Check sheet for the modelled part. Datum: model origin and axes. Units: mm. A direction names the side the tool comes from. Give positions to 0.01 mm unless a question says otherwise; leave off trailing zeros. Write each loop counter-clockwise with the first axis right and the second up, starting at its lowest first coordinate (ties: lowest second). Pieces come first, ordered by that corner, then holes. Notation, with made-up numbers: (67, 10) -> (81, 10) arc R27 cw to (81, 29) -> close; hole circle Ø3 at (4.5, 16.5). An arc over 180 degrees is marked (long way). Answer as a JSON object with one key per item and string values.
from build123d import *

# Parameters (mm, degrees)
F0_W          = 125
F0_H          = 40
F0_R          = 5
F1_DEPTH      = 25
F2_R          = 11
F3_DEPTH      = 10
F4_W          = 40
F4_H          = 25
F5_DEPTH      = 25
F6_R          = 4.25
F7_DEPTH      = 40
F9_DEPTH      = 6
F10_T4_DEPTH  = 25
F10_T10_DEPTH = 25
F10_T16_DEPTH = 25
F10_T23_DEPTH = 25
F10_T29_DEPTH = 25
F10_T35_DEPTH = 25
F10_T41_DEPTH = 25
F10_T47_DEPTH = 25
F10_T54_DEPTH = 25
F10_T60_DEPTH = 25
F10_T63_DEPTH = 50


# Not quite as in the source:
# - a fillet or chamfer that OpenCascade refuses, or shapes differently, is made with other operations: its cross-section is extruded or revolved along the edge and cut away or added


with BuildPart() as f1:
    # F0 (on Front) → F1 (new body)
    with BuildSketch(Plane.XZ):
        with Locations((-7.5, 0)):
            Rectangle(F0_W, F0_H)
        with Locations((-50, 0)):
            Circle(F0_R, mode=Mode.SUBTRACT)
        Circle(F0_R, mode=Mode.SUBTRACT)
        with Locations((40, 0)):
            Circle(F0_R, mode=Mode.SUBTRACT)
    extrude(amount=F1_DEPTH)

    # F2 (on face) → F3 (cut)
    with BuildSketch(Plane.XZ.offset(25)):
        with Locations((-50, 0)):
            Circle(F2_R)
        Circle(F2_R)
        with Locations((40, 0)):
            Circle(F2_R)
    extrude(amount=-F3_DEPTH, mode=Mode.SUBTRACT)

    # F4 (on face) → F5 (join)
    with BuildSketch(Plane(origin=(0, 0, 0), x_dir=(-1, 0, 0), z_dir=(0, 1, 0))):
        with Locations((50, 32.5)):
            Rectangle(F4_W, F4_H)
        with Locations((50, -32.5)):
            Rectangle(F4_W, F4_H)
    extrude(amount=-F5_DEPTH)

    # F6 (on face) → F7 (cut, through all)
    with BuildSketch(Plane(origin=(-70, 0, 0), x_dir=(0, -1, 0), z_dir=(-1, 0, 0))):
        with Locations((12.5, 27.5)):
            Circle(F6_R)
        with Locations((12.5, -27.5)):
            Circle(F6_R)
    extrude(amount=-F7_DEPTH, mode=Mode.SUBTRACT)

    # F8 (on face) → F9 (cut)
    with BuildSketch(Plane.YZ.offset(-30)):
        Polygon((-8.4585481157, 34.5), (-16.5414518843, 34.5), (-20.5829037687, 27.5), (-16.5414518843, 20.5), (-8.4585481157, 20.5), (-4.4170962313, 27.5), align=None)
        Polygon((-8.4585481157, -20.5), (-16.5414518843, -20.5), (-20.5829037687, -27.5), (-16.5414518843, -34.5), (-8.4585481157, -34.5), (-4.4170962313, -27.5), align=None)
    extrude(amount=-F9_DEPTH, mode=Mode.SUBTRACT)

    # F10: fillet of radius 5 on 6 edges, made by hand


with BuildPart() as f10_tool2:
    # F10_s3 → F10_t4 (new body)
    with BuildSketch(Plane.XZ):
        with BuildLine():
            ThreePointArc((-25, 20), (-28.5355339059, 21.4644660941), (-30, 25))
            Line((-30, 25), (-30, 20))
            Line((-30, 20), (-25, 20))
        make_face()
    extrude(amount=F10_T4_DEPTH)

    split(bisect_by=Plane.XY.offset(20.5), keep=Keep.BOTTOM)

    split(bisect_by=Plane(origin=(0, -15.2206714755, 8.7876587737), x_dir=(1, 0, 0), z_dir=(0, 0.8660254038, -0.5)), keep=Keep.TOP)


with BuildPart() as f1_1:
    add(f1.part)

    # F10_t1: union F10_tool2
    add(f10_tool2.part)


with BuildPart() as f10_tool8:
    # F10_s9 → F10_t10 (new body)
    with BuildSketch(Plane.XZ):
        with BuildLine():
            ThreePointArc((-25, 20), (-28.5355339059, 21.4644660941), (-30, 25))
            Line((-30, 25), (-30, 20))
            Line((-30, 20), (-25, 20))
        make_face()
    extrude(amount=F10_T10_DEPTH)

    split(bisect_by=Plane.XY.offset(20.5), keep=Keep.TOP)

    split(bisect_by=Plane(origin=(0, -15.2206714755, 8.7876587737), x_dir=(1, 0, 0), z_dir=(0, 0.8660254038, -0.5)), keep=Keep.TOP)


with BuildPart() as f1_2:
    add(f1_1.part)

    # F10_t7: union F10_tool8
    add(f10_tool8.part)


with BuildPart() as f10_tool14:
    # F10_s15 → F10_t16 (new body)
    with BuildSketch(Plane.XZ):
        with BuildLine():
            ThreePointArc((-25, 20), (-28.5355339059, 21.4644660941), (-30, 25))
            Line((-30, 25), (-30, 20))
            Line((-30, 20), (-25, 20))
        make_face()
    extrude(amount=F10_T16_DEPTH)

    split(bisect_by=Plane(origin=(0, -3.5293285245, -2.0376587737), x_dir=(1, 0, 0), z_dir=(0, 0.8660254038, 0.5)), keep=Keep.TOP)

    split(bisect_by=Plane.XY.offset(20.5), keep=Keep.BOTTOM)

    split(bisect_by=Plane(origin=(0, -15.2206714755, 8.7876587737), x_dir=(1, 0, 0), z_dir=(0, -0.8660254038, 0.5)), keep=Keep.TOP)


with BuildPart() as f1_3:
    add(f1_2.part)

    # F10_t13: union F10_tool14
    add(f10_tool14.part)


with BuildPart() as f10_tool21:
    # F10_s22 → F10_t23 (new body)
    with BuildSketch(Plane.XZ):
        with BuildLine():
            ThreePointArc((-25, 20), (-28.5355339059, 21.4644660941), (-30, 25))
            Line((-30, 25), (-30, 20))
            Line((-30, 20), (-25, 20))
        make_face()
    extrude(amount=F10_T23_DEPTH)

    split(bisect_by=Plane(origin=(0, -3.5293285245, -2.0376587737), x_dir=(1, 0, 0), z_dir=(0, -0.8660254038, -0.5)), keep=Keep.TOP)

    split(bisect_by=Plane.XY.offset(20.5), keep=Keep.BOTTOM)


with BuildPart() as f1_4:
    add(f1_3.part)

    # F10_t20: union F10_tool21
    add(f10_tool21.part)


with BuildPart() as f10_tool27:
    # F10_s28 → F10_t29 (new body)
    with BuildSketch(Plane.XZ):
        with BuildLine():
            ThreePointArc((-25, 20), (-28.5355339059, 21.4644660941), (-30, 25))
            Line((-30, 25), (-30, 20))
            Line((-30, 20), (-25, 20))
        make_face()
    extrude(amount=F10_T29_DEPTH)

    split(bisect_by=Plane(origin=(0, -3.5293285245, -2.0376587737), x_dir=(1, 0, 0), z_dir=(0, -0.8660254038, -0.5)), keep=Keep.TOP)

    split(bisect_by=Plane.XY.offset(20.5), keep=Keep.TOP)


with BuildPart() as f1_5:
    add(f1_4.part)

    # F10_t26: union F10_tool27
    add(f10_tool27.part)


with BuildPart() as f10_tool33:
    # F10_s34 → F10_t35 (new body)
    with BuildSketch(Plane.XZ):
        with BuildLine():
            ThreePointArc((-25, -20), (-28.5355339059, -21.4644660941), (-30, -25))
            Line((-30, -25), (-30, -20))
            Line((-30, -20), (-25, -20))
        make_face()
    extrude(amount=F10_T35_DEPTH)

    split(bisect_by=Plane.XY.offset(-20.5), keep=Keep.TOP)

    split(bisect_by=Plane(origin=(0, -15.2206714755, -8.7876587737), x_dir=(1, 0, 0), z_dir=(0, 0.8660254038, 0.5)), keep=Keep.TOP)


with BuildPart() as f1_6:
    add(f1_5.part)

    # F10_t32: union F10_tool33
    add(f10_tool33.part)


with BuildPart() as f10_tool39:
    # F10_s40 → F10_t41 (new body)
    with BuildSketch(Plane.XZ):
        with BuildLine():
            ThreePointArc((-25, -20), (-28.5355339059, -21.4644660941), (-30, -25))
            Line((-30, -25), (-30, -20))
            Line((-30, -20), (-25, -20))
        make_face()
    extrude(amount=F10_T41_DEPTH)

    split(bisect_by=Plane.XY.offset(-20.5), keep=Keep.BOTTOM)

    split(bisect_by=Plane(origin=(0, -15.2206714755, -8.7876587737), x_dir=(1, 0, 0), z_dir=(0, 0.8660254038, 0.5)), keep=Keep.TOP)


with BuildPart() as f1_7:
    add(f1_6.part)

    # F10_t38: union F10_tool39
    add(f10_tool39.part)


with BuildPart() as f10_tool45:
    # F10_s46 → F10_t47 (new body)
    with BuildSketch(Plane.XZ):
        with BuildLine():
            ThreePointArc((-25, -20), (-28.5355339059, -21.4644660941), (-30, -25))
            Line((-30, -25), (-30, -20))
            Line((-30, -20), (-25, -20))
        make_face()
    extrude(amount=F10_T47_DEPTH)

    split(bisect_by=Plane.XY.offset(-20.5), keep=Keep.TOP)

    split(bisect_by=Plane(origin=(0, -3.5293285245, 2.0376587737), x_dir=(1, 0, 0), z_dir=(0, 0.8660254038, -0.5)), keep=Keep.TOP)

    split(bisect_by=Plane(origin=(0, -15.2206714755, -8.7876587737), x_dir=(1, 0, 0), z_dir=(0, -0.8660254038, -0.5)), keep=Keep.TOP)


with BuildPart() as f1_8:
    add(f1_7.part)

    # F10_t44: union F10_tool45
    add(f10_tool45.part)


with BuildPart() as f10_tool52:
    # F10_s53 → F10_t54 (new body)
    with BuildSketch(Plane.XZ):
        with BuildLine():
            ThreePointArc((-25, -20), (-28.5355339059, -21.4644660941), (-30, -25))
            Line((-30, -25), (-30, -20))
            Line((-30, -20), (-25, -20))
        make_face()
    extrude(amount=F10_T54_DEPTH)

    split(bisect_by=Plane.XY.offset(-20.5), keep=Keep.TOP)

    split(bisect_by=Plane(origin=(0, -3.5293285245, 2.0376587737), x_dir=(1, 0, 0), z_dir=(0, -0.8660254038, 0.5)), keep=Keep.TOP)


with BuildPart() as f1_9:
    add(f1_8.part)

    # F10_t51: union F10_tool52
    add(f10_tool52.part)


with BuildPart() as f10_tool58:
    # F10_s59 → F10_t60 (new body)
    with BuildSketch(Plane.XZ):
        with BuildLine():
            ThreePointArc((-25, -20), (-28.5355339059, -21.4644660941), (-30, -25))
            Line((-30, -25), (-30, -20))
            Line((-30, -20), (-25, -20))
        make_face()
    extrude(amount=F10_T60_DEPTH)

    split(bisect_by=Plane.XY.offset(-20.5), keep=Keep.BOTTOM)

    split(bisect_by=Plane(origin=(0, -3.5293285245, 2.0376587737), x_dir=(1, 0, 0), z_dir=(0, -0.8660254038, 0.5)), keep=Keep.TOP)


with BuildPart() as f1_10:
    add(f1_9.part)

    # F10_t57: union F10_tool58
    add(f10_tool58.part)

    # F10_s64 → F10_t63 (cut)
    with BuildSketch(Plane.XZ.offset(-12.5)):
        with BuildLine():
            ThreePointArc((-35, 45), (-31.4644660941, 43.5355339059), (-30, 40))
            Line((-30, 40), (-30, 45))
            Line((-30, 45), (-35, 45))
        make_face()
        with BuildLine():
            ThreePointArc((-30, -40), (-31.4644660941, -43.5355339059), (-35, -45))
            Line((-35, -45), (-30, -45))
            Line((-30, -45), (-30, -40))
        make_face()
        with BuildLine():
            ThreePointArc((55, -15), (53.5355339059, -18.5355339059), (50, -20))
            Line((50, -20), (55, -20))
            Line((55, -20), (55, -15))
        make_face()
        with BuildLine():
            ThreePointArc((55, 15), (53.5355339059, 18.5355339059), (50, 20))
            Line((50, 20), (55, 20))
            Line((55, 20), (55, 15))
        make_face()
    extrude(amount=F10_T63_DEPTH, mode=Mode.SUBTRACT)


solid = f1_10.part
1. Sectioned sample at D-D, the plane x = 40. Enter the section's corners in (y, z).
Determined:
{"outline": "(-25, -20) -> (0, -20) -> (0, -5) -> (-15, -5) -> (-15, -11) -> (-25, -11) -> close; (-25, 11) -> (-15, 11) -> (-15, 5) -> (0, 5) -> (0, 20) -> (-25, 20) -> close"}
2. Sectioned sample at C-C, the plane y = -12.75. State how many separate pieces and enclosed holes the cut face has, plus the area to 3 significant figures.
Determined:
{"separate pieces": "3", "enclosed holes": "3", "area": "6,000 mm^2"}
3. Go/stop test with flat-tipped pins: P1, Ø9, axis at x = -50, z = 0, coming from the -Y side; P2, Ø7.5, axis at y = -15, z = 31.5, coming from the +X side; P3, Ø2.5, axis at x = -29.5, y = -14, coming from the +Z side; P4, Ø1.5, axis at x = 9.5, y = -2.5, coming from the +Z side. Record where each tip stops, or that it passes through.
Determined:
{"P1": "through", "P2": "x = -30", "P3": "z = 42.63", "P4": "z = 20"}
4. Sectioned sample at B-B, the plane z = 0. Enter the section's corners in (x, y), plus the area to 4 significant figures.
Determined:
{"outline": "(-70, -25) -> (-61, -25) -> (-61, -15) -> (-55, -15) -> (-55, 0) -> (-70, 0) -> close; (-45, -15) -> (-39, -15) -> (-39, -25) -> (-11, -25) -> (-11, -15) -> (-5, -15) -> (-5, 0) -> (-45, 0) -> close; (5, -15) -> (11, -15) -> (11, -25) -> (29, -25) -> (29, -15) -> (35, -15) -> (35, 0) -> (5, 0) -> close; (45, -15) -> (51, -15) -> (51, -25) -> (55, -25) -> (55, 0) -> (45, 0) -> close", "area": "2,015 mm^2"}
5. Mould release check, pull along Z, two halves, no side actions. Record for faces 5 (the face through (-53.238, -14.785, -23.916)), 6 (the face through (12, -12, 20)), 7 (the face through (-31, -12, -43)): released by +Z, released by -Z, zero draft, split by the parting line, or undercut.
Determined:
{"face 5": "undercut", "face 6": "released by +Z", "face 7": "released by -Z"}
6. Access from +Z, -Z, +X, -X, +Y, -Y to the whole of each face (thin tool, end or side, straight path). Record for faces 1 (the face through (-21, 0, 1)), 2 (the face through (-32.958, -6.466, -31.049)), 3 (the face through (12, -12, -20)), 4 (the face through (2, -15, -5)).
Determined:
{"face 1": "+Z, -Z, +X, -X, +Y", "face 2": "+X", "face 3": "-Z, +X, +Y, -Y", "face 4": "-Y"}
7. Scan lines: L1, parallel to Z at x = -57, y = -12.75; L2, parallel to X at y = -8.25, z = 0; L3, parallel to Z at x = -50, y = -12.5. Record each from-to range of solid material in increasing order. Write a range as [from, to].
Determined:
{"L1": "[-45, -31.74], [-23.26, 23.26], [31.74, 45]", "L2": "[-70, -55], [-45, -5], [5, 35], [45, 55]", "L3": "[-45, -31.75], [-23.25, -5], [5, 23.25], [31.75, 45]"}
8. Sectioned sample at A-A, the plane x = -50. Enter the section's corners in (y, z), plus the area to 3 significant figures.
Determined:
{"outline": "(-25, -45) -> (0, -45) -> (0, -5) -> (-15, -5) -> (-15, -11) -> (-25, -11) -> close; (-25, 11) -> (-15, 11) -> (-15, 5) -> (0, 5) -> (0, 45) -> (-25, 45) -> close; hole circle Ø8.5 at (-12.5, -27.5); hole circle Ø8.5 at (-12.5, 27.5)", "area": "1,770 mm^2"}
